Verification items for the finished model (mm, model axes). A direction names the side the tool comes from. Round coordinates to 2 decimals unless told otherwise and drop trailing zeros. Write each loop counter-clockwise with the first axis right and the second up, starting at its lowest first coordinate (ties: lowest second). Pieces come first, ordered by that corner, then holes. Notation, with made-up numbers: M -39,-13.75 L -6,-13.75 A15 ccw -6,2.25 Z; hole C 83.25,-30.5 d1. An arc over 180 degrees is marked long. One line per item, written item: value. Start each with the question number.
Item 1: Gauge pin test, flat end, axial feed: pin 1 (1.2 mm diameter, centred on y = 0.5, z = -64, fed in from -X). Record the tip position at first contact, or that the pin passes through.
Item 2: Tool access check on faces 4 (the face through (22.153, 0, 2)), 5 (the face through (11, 0, -43.251)), 6 (the face through (40, 1.191, -14)). Record the directions out of +Z, -Z, +X, -X, +Y, -Y that give a thin tool (end or side, any length) a straight path to the whole face; none if there is none.
Item 3: Section check D-D, the plane y = -0.65. State how many separate pieces and enclosed holes the cut face has, then the cut area to 3 significant figures.
Item 4: Section check C-C, the plane z = 30. Record the cut outline in (x, y), then the cut area to 3 significant figures.
Item 5: Thickness scan on probe 1 along Z at (x, y) = (31, -0.5); probe 2 along X at (y, z) = (0.1, 25.5); probe 3 along X at (y, z) = (-0.9, -23.5). Record the ranges inside material, lowest first. Write a range as from..to.
Item 6: Section check B-B, the plane z = -31.5. Record the cut outline in (x, y).
Item 7: Section check A-A, the plane z = 2.5. Record the cut outline in (x, y), then the cut area to 3 significant figures.
Item 8: Draft check along X on faces 1 (the face through (25.109, 0, -24)), 2 (the face through (48.149, 0, 33)), 3 (the face through (50, 0, 5.167)). Enter one of: +X half, -X half, draft (parallel to the pull), parting line (faces both ways), or undercut.
from build123d import *

# Parameters (mm, degrees)
SKETCH1_W           = 17.065625
SKETCH1_H           = 9.525
SKETCH1_R           = 1.5875
BOSS_EXTRUDE2_DEPTH = 1.190625


with BuildPart() as part:
    # Sketch1 → Boss-Extrude2 (new, symmetric)
    with BuildSketch(Plane(origin=(0, 0, 0), x_dir=(1, 0, 0), z_dir=(0, 1, 0))):
        Polygon((48.148623935, -59.93613473), (48.148623935, -5.16738473), (51.819717685, -5.16738473), (51.819717685, 43.25136527), (48.049405185, 43.25136527), (48.049405185, 85.71699027), (13.322842685, 85.71699027), (13.322842685, 43.25136527), (9.552530185, 43.25136527), (9.552530185, -5.16738473), (13.223623935, -5.16738473), (13.223623935, -59.93613473), align=None)
        with Locations((30.686123935, 12.29511527)):
            Rectangle(SKETCH1_W, SKETCH1_H, mode=Mode.SUBTRACT)
        with Locations((30.686123935, -1.99238473)):
            Rectangle(SKETCH1_W, SKETCH1_H, mode=Mode.SUBTRACT)
        with BuildLine():
            Line((16.398623935, -24.61425973), (16.398623935, -33.74238473))
            ThreePointArc((16.398623935, -33.74238473), (15.604873935, -34.53613473), (14.811123935, -33.74238473))
            Line((14.811123935, -33.74238473), (14.811123935, -24.61425973))
            ThreePointArc((14.811123935, -24.61425973), (15.604873935, -23.82050973), (16.398623935, -24.61425973))
        make_face(mode=Mode.SUBTRACT)
        with Locations(Location((18.978311435, -18.66113473, 0), (0, 0, 90))):
            Circle(SKETCH1_R, mode=Mode.SUBTRACT)
        with Locations(Location((18.978311435, -6.75488473, 0), (0, 0, 90))):
            Circle(SKETCH1_R, mode=Mode.SUBTRACT)
        with BuildLine():
            ThreePointArc((23.343936435, -23.42363473), (22.153311435, -22.23300973), (23.343936435, -21.04238473))
            Line((23.343936435, -21.04238473), (38.028311435, -21.04238473))
            ThreePointArc((38.028311435, -21.04238473), (39.218936435, -22.23300973), (38.028311435, -23.42363473))
            Line((38.028311435, -23.42363473), (23.343936435, -23.42363473))
        make_face(mode=Mode.SUBTRACT)
        with BuildLine():
            ThreePointArc((46.561123935, -33.74238473), (45.767373935, -34.53613473), (44.973623935, -33.74238473))
            Line((44.973623935, -33.74238473), (44.973623935, -24.61425973))
            ThreePointArc((44.973623935, -24.61425973), (45.767373935, -23.82050973), (46.561123935, -24.61425973))
            Line((46.561123935, -24.61425973), (46.561123935, -33.74238473))
        make_face(mode=Mode.SUBTRACT)
        with Locations(Location((42.393936435, -18.66113473, 0), (0, 0, 90))):
            Circle(SKETCH1_R, mode=Mode.SUBTRACT)
        with Locations(Location((42.393936435, -6.75488473, 0), (0, 0, 90))):
            Circle(SKETCH1_R, mode=Mode.SUBTRACT)
        with BuildLine():
            ThreePointArc((15.108780185, -4.37363473), (14.315030185, -5.16738473), (13.521280185, -4.37363473))
            Line((13.521280185, -4.37363473), (13.521280185, 37.69511527))
            ThreePointArc((13.521280185, 37.69511527), (14.315030185, 38.48886527), (15.108780185, 37.69511527))
            Line((15.108780185, 37.69511527), (15.108780185, -4.37363473))
        make_face(mode=Mode.SUBTRACT)
        with Locations(Location((18.978311435, 17.65292777, 0), (0, 0, 90))):
            Circle(SKETCH1_R, mode=Mode.SUBTRACT)
        with BuildLine():
            Line((26.696280185, 25.590053861), (26.696280185, 21.82011527))
            ThreePointArc((26.696280185, 21.82011527), (25.902530185, 21.02636527), (25.108780185, 21.82011527))
            Line((25.108780185, 21.82011527), (25.108780185, 25.590053861))
            ThreePointArc((25.108780185, 25.590053861), (25.902530185, 26.383803861), (26.696280185, 25.590053861))
        make_face(mode=Mode.SUBTRACT)
        with BuildLine():
            Line((26.696280185, 33.328742451), (26.696280185, 29.558803861))
            ThreePointArc((26.696280185, 29.558803861), (25.902530185, 28.765053861), (25.108780185, 29.558803861))
            Line((25.108780185, 29.558803861), (25.108780185, 33.328742451))
            ThreePointArc((25.108780185, 33.328742451), (25.902530185, 34.122492451), (26.696280185, 33.328742451))
        make_face(mode=Mode.SUBTRACT)
        with BuildLine():
            ThreePointArc((46.263467685, 37.69511527), (47.057217685, 38.48886527), (47.850967685, 37.69511527))
            Line((47.850967685, 37.69511527), (47.850967685, -4.37363473))
            ThreePointArc((47.850967685, -4.37363473), (47.057217685, -5.16738473), (46.263467685, -4.37363473))
            Line((46.263467685, -4.37363473), (46.263467685, 37.69511527))
        make_face(mode=Mode.SUBTRACT)
        with Locations(Location((42.393936435, 17.65292777, 0), (0, 0, 90))):
            Circle(SKETCH1_R, mode=Mode.SUBTRACT)
        with BuildLine():
            ThreePointArc((36.263467685, 21.82011527), (35.469717685, 21.02636527), (34.675967685, 21.82011527))
            Line((34.675967685, 21.82011527), (34.675967685, 25.590053861))
            ThreePointArc((34.675967685, 25.590053861), (35.469717685, 26.383803861), (36.263467685, 25.590053861))
            Line((36.263467685, 25.590053861), (36.263467685, 21.82011527))
        make_face(mode=Mode.SUBTRACT)
        with BuildLine():
            ThreePointArc((36.263467685, 29.558803861), (35.469717685, 28.765053861), (34.675967685, 29.558803861))
            Line((34.675967685, 29.558803861), (34.675967685, 33.328742451))
            ThreePointArc((34.675967685, 33.328742451), (35.469717685, 34.122492451), (36.263467685, 33.328742451))
            Line((36.263467685, 33.328742451), (36.263467685, 29.558803861))
        make_face(mode=Mode.SUBTRACT)
    extrude(amount=BOSS_EXTRUDE2_DEPTH, both=True)


solid = part.part
Response values:
1. pin 1: stops at x = 13.32
2. face 4: +Y, -Y
2. face 5: -Z, -X, +Y, -Y
2. face 6: +Z, -Z, +X, -X, +Y
3. separate pieces: 1
3. enclosed holes: 17
3. area: 4,820 mm2
4. outline: M 13.22,-1.19 L 14.81,-1.19 L 14.81,1.19 L 13.22,1.19 Z; M 16.4,-1.19 L 44.97,-1.19 L 44.97,1.19 L 16.4,1.19 Z; M 46.56,-1.19 L 48.15,-1.19 L 48.15,1.19 L 46.56,1.19 Z
4. area: 75.6 mm2
5. probe 1: z = -85.72..-17.06, -7.53..-2.77, 6.75..21.04, 23.42..59.94
5. probe 2: x = 13.22..14.81, 16.4..44.97, 46.56..48.15
5. probe 3: x = 9.55..13.52, 15.11..25.11, 26.7..34.68, 36.26..46.26, 47.85..51.82
6. outline: M 9.55,-1.19 L 13.52,-1.19 L 13.52,1.19 L 9.55,1.19 Z; M 15.11,-1.19 L 25.11,-1.19 L 25.11,1.19 L 15.11,1.19 Z; M 26.7,-1.19 L 34.68,-1.19 L 34.68,1.19 L 26.7,1.19 Z; M 36.26,-1.19 L 46.26,-1.19 L 46.26,1.19 L 36.26,1.19 Z; M 47.85,-1.19 L 51.82,-1.19 L 51.82,1.19 L 47.85,1.19 Z
7. outline: M 9.55,-1.19 L 13.52,-1.19 L 13.52,1.19 L 9.55,1.19 Z; M 15.11,-1.19 L 22.15,-1.19 L 22.15,1.19 L 15.11,1.19 Z; M 39.22,-1.19 L 46.26,-1.19 L 46.26,1.19 L 39.22,1.19 Z; M 47.85,-1.19 L 51.82,-1.19 L 51.82,1.19 L 47.85,1.19 Z
7. area: 52.5 mm2
8. face 1: undercut
8. face 2: +X half
8. face 3: draft
